```python
from build123d import *

# Parameters (mm, degrees)
EXTRUDE_1_DEPTH = 2.5


with BuildPart() as part:
    # 草图1 → 凸台-拉伸1 (new body)
    with BuildSketch(Plane.XY):
        with BuildLine():
            Line((7.183350415, -12.48442441), (7.183350415, 22.607248677))
            ThreePointArc((7.183350415, 22.607248677), (6.451117367, 24.37501563), (4.683350415, 25.107248677))
            Line((4.683350415, 25.107248677), (-4.316649585, 25.107248677))
            ThreePointArc((-4.316649585, 25.107248677), (-6.084416538, 24.37501563), (-6.816649585, 22.607248677))
            Line((-6.816649585, 22.607248677), (-6.816649585, -12.48442441))
            ThreePointArc((-6.816649585, -12.48442441), (-6.889401362, -13.018946893), (-7.102363871, -13.514581917))
            ThreePointArc((-7.102363871, -13.514581917), (0.183350415, -26.392751323), (7.4690647, -13.514581917))
            ThreePointArc((7.4690647, -13.514581917), (7.256102191, -13.018946893), (7.183350415, -12.48442441))
        make_face()
        with BuildLine():
            Line((4.341271874, -19.600508074), (4.124778706, -19.475515685))
            ThreePointArc((4.124778706, -19.475515685), (3.994781084, -19.323417542), (3.98933022, -19.123408756))
            ThreePointArc((3.98933022, -19.123408756), (3.64745203, -15.892751323), (1.020559717, -13.981347408))
            ThreePointArc((1.020559717, -13.981347408), (0.850072459, -13.876622428), (0.783350415, -13.687992114))
            Line((0.783350415, -13.687992114), (0.783350415, -13.438007336))
            ThreePointArc((0.783350415, -13.438007336), (0.183350415, -12.838007336), (-0.416649585, -13.438007336))
            Line((-0.416649585, -13.438007336), (-0.416649585, -13.687992114))
            ThreePointArc((-0.416649585, -13.687992114), (-0.48337163, -13.876622428), (-0.653858888, -13.981347408))
            ThreePointArc((-0.653858888, -13.981347408), (-3.280751201, -15.892751323), (-3.622629391, -19.123408756))
            ThreePointArc((-3.622629391, -19.123408756), (-3.628080255, -19.323417542), (-3.758077877, -19.475515685))
            Line((-3.758077877, -19.475515685), (-3.974571045, -19.600508074))
            ThreePointArc((-3.974571045, -19.600508074), (-4.194186288, -20.420123316), (-3.374571045, -20.639738558))
            Line((-3.374571045, -20.639738558), (-3.158077877, -20.514746169))
            ThreePointArc((-3.158077877, -20.514746169), (-2.961358211, -20.478213997), (-2.785420089, -20.573497804))
            ThreePointArc((-2.785420089, -20.573497804), (0.183350415, -21.892751323), (3.152120918, -20.573497804))
            ThreePointArc((3.152120918, -20.573497804), (3.32805904, -20.478213997), (3.524778706, -20.514746169))
            Line((3.524778706, -20.514746169), (3.741271874, -20.639738558))
            ThreePointArc((3.741271874, -20.639738558), (4.560887117, -20.420123316), (4.341271874, -19.600508074))
        make_face(mode=Mode.SUBTRACT)
        with BuildLine():
            ThreePointArc((2.483350415, -1.892751323), (0.183350415, 0.407248677), (-2.116649585, -1.892751323))
            ThreePointArc((-2.116649585, -1.892751323), (0.183350415, -4.192751323), (2.483350415, -1.892751323))
        make_face(mode=Mode.SUBTRACT)
        with BuildLine():
            ThreePointArc((2.483350415, 18.107248677), (0.183350415, 20.407248677), (-2.116649585, 18.107248677))
            ThreePointArc((-2.116649585, 18.107248677), (0.183350415, 15.807248677), (2.483350415, 18.107248677))
        make_face(mode=Mode.SUBTRACT)
    extrude(amount=EXTRUDE_1_DEPTH)


solid = part.part
```
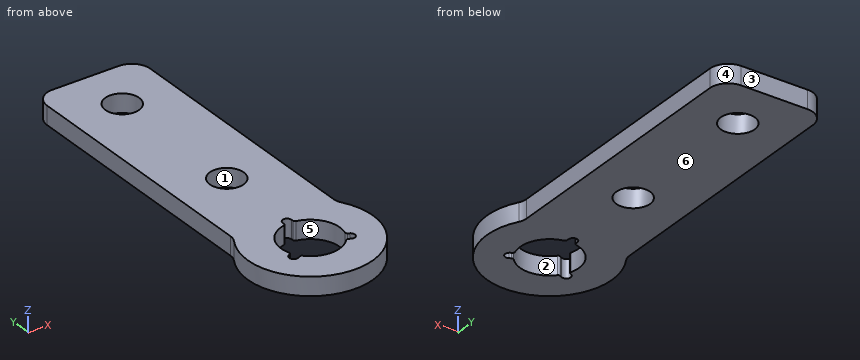
Read the model definition and answer for the solid it produces. Units are mm, in the model's axes. Face numbers are marked on the shaded views. A direction names the side the tool comes from. Give positions to 0.01 mm unless a question says otherwise; leave off trailing zeros. Order: outer loops, then holes, each group sorted by start corner. A loop starts at its lowest first (then second) coordinate and runs counter-clockwise, first axis right, second up.
(1) Straight lines are drawn through the part: L1, parallel to X at y = -13.5, z = 1.5; L2, parallel to X at y = -2, z = 1.75; L3, parallel to Y at x = 1.5, z = 1.75. For each, find the intervals that lie inside material, in ascending order.
(2) Find section C-C (y = -17.5). Give the vertices of the cut face in (x, z), plus the area to 3 significant figures.
(3) Given pin 1 (1 mm diameter, centred on y = -4.5, z = 1.5, fed in from +X), flat-ended and moving along its own axis, determine where the tip first touches the part or whether it passes through.
(4) Find section D-D (x = -6). Give the vertices of the cut face in (y, z), plus the area to 3 significant figures.
(5) Find section A-A (x = 0.25). Give the vertices of the cut face in (y, z).
(6) For the marked faces 5 and 6, determine the directions among +Z, -Z, +X, -X, +Y, -Y from which every point of the face is accessible in a straight line to the end or side of a thin tool.
(7) For a pull along X with two mould halves and no side action, classify the marked faces 1, 2, 3 and 4 as released by +X, released by -X, zero draft, split by the parting line, or undercut.
(8) Find section B-B (z = 1.1). Give the vertices of the cut face in (x, y).
Result sheet:
1. L1: x = -7.09 to -0.42, 0.78 to 7.46
1. L2: x = -6.82 to -2.11, 2.48 to 7.18
1. L3: y = -26.29 to -21.67, -14.12 to -3.78, -0.01 to 16.22, 19.99 to 25.11
2. outline: (-8.31, 0) - (-3.8, 0) - (-3.8, 2.5) - (-8.31, 2.5) - close; (4.16, 0) - (8.67, 0) - (8.67, 2.5) - (4.16, 2.5) - close
2. area: 22.6 mm2
3. pin 1: stops at x = 7.18
4. outline: (-23.73, 0) - (24.46, 0) - (24.46, 2.5) - (-23.73, 2.5) - close
4. area: 120 mm2
5. outline: (-26.39, 0) - (-21.89, 0) - (-21.89, 2.5) - (-26.39, 2.5) - close; (-12.84, 0) - (-4.19, 0) - (-4.19, 2.5) - (-12.84, 2.5) - close; (0.41, 0) - (15.81, 0) - (15.81, 2.5) - (0.41, 2.5) - close; (20.41, 0) - (25.11, 0) - (25.11, 2.5) - (20.41, 2.5) - close
6. face 5: +Z, -Z
6. face 6: -Z, +X, -X, +Y, -Y
7. face 1: undercut
7. face 2: undercut
7. face 3: zero draft
7. face 4: released by +X
8. outline: (-7.1, -13.51) arc R8.5 ccw (long way) to (7.47, -13.51) arc R2 cw to (7.18, -12.48) - (7.18, 22.61) arc R2.5 ccw to (4.68, 25.11) - (-4.32, 25.11) arc R2.5 ccw to (-6.82, 22.61) - (-6.82, -12.48) arc R2 cw to start; hole (-3.97, -19.6) arc R0.6 ccw to (-3.37, -20.64) - (-3.16, -20.51) arc R0.3 cw to (-2.79, -20.57) arc R4 ccw to (3.15, -20.57) arc R0.3 cw to (3.52, -20.51) - (3.74, -20.64) arc R0.6 ccw to (4.34, -19.6) - (4.12, -19.48) arc R0.3 cw to (3.99, -19.12) arc R4 ccw to (1.02, -13.98) arc R0.3 cw to (0.78, -13.69) - (0.78, -13.44) arc R0.6 ccw to (-0.42, -13.44) - (-0.42, -13.69) arc R0.3 cw to (-0.65, -13.98) arc R4 ccw to (-3.62, -19.12) arc R0.3 cw to (-3.76, -19.48) - close; hole circle Ø4.6 at (0.18, -1.89); hole circle Ø4.6 at (0.18, 18.11)
